The model under review builds one solid part; all positions refer to its coordinate system, in mm. A direction names the side the tool comes from. Round coordinates to 2 decimals unless told otherwise and drop trailing zeros. Order: outer loops, then holes, each group sorted by start corner. A loop starts at its lowest first (then second) coordinate and runs counter-clockwise, first axis right, second up.
Solid Edge part; units mm, degrees
sketch "Sketch1" plane through (0, 0, 0) normal (0, 0, 1) x (1, 0, 0)
  line L0 (-120, -60) -> (120, -60)
  line L1 (120, 120) -> (120, -60)
  line L2 (120, 120) -> (-120, 120)
  line L3 (-120, 120) -> (-120, -60)
extrude "Protrusion1" add sketch "Sketch1" along normal mid plane 50
fillet "Round_1" radius 30 4 edges at (-120, 120, 0) (-120, -60, 0) (120, -60, 0) (120, 120, 0)
hole "Hole_6" at (83, -30, -25) direction (0, 0, 1) diameter 4.917 depth 21
hole "Hole1" at (83, 30, -25) direction (0, 0, 1) diameter 4.917 depth 21
hole "Hole2" at (-83, 30, -25) direction (0, 0, 1) diameter 4.917 depth 21
hole "Hole3" at (-83, -30, -25) direction (0, 0, 1) diameter 4.917 depth 21
(1) Consider section B-B (x = 83). Write out the cut boundary in (y, z).
Data:
outline: (-60, -25) - (-32.46, -25) - (-32.46, -4) - (-27.54, -4) - (-27.54, -25) - (27.54, -25) - (27.54, -4) - (32.46, -4) - (32.46, -25) - (120, -25) - (120, 25) - (-60, 25) - close
(2) For faces 4 (the cylindrical face through (85.4, -30.53, -14.35)), 5 (the cylindrical face through (-111.445, 110.979, -0.35)), list the 3-axis set-ups (+Z, -Z, +X, -X, +Y, -Y) from which the entire face can be reached by the end or side of a thin tool; tool diameter is ignored.
Data:
face 4: -Z
face 5: +Z, -Z, -X, +Y
(3) Consider section D-D (y = -43). Write out the cut boundary in (x, z), and give its area (3 significant figures).
Data:
outline: (-117.04, -25) - (117.04, -25) - (117.04, 25) - (-117.04, 25) - close
area: 11,700 mm2
(4) Consider section C-C (z = -16). Write out the cut boundary in (x, y), and give its area (3 significant figures).
Data:
outline: (-120, -30) arc R30 ccw to (-90, -60) - (90, -60) arc R30 ccw to (120, -30) - (120, 90) arc R30 ccw to (90, 120) - (-90, 120) arc R30 ccw to (-120, 90) - close; hole circle Ø4.92 at (-83, -30); hole circle Ø4.92 at (-83, 30); hole circle Ø4.92 at (83, -30); hole circle Ø4.92 at (83, 30)
area: 42,400 mm2
(5) Consider section A-A (y = 30). Write out the cut boundary in (x, z), and give its area (3 significant figures).
Data:
outline: (-120, -25) - (-85.46, -25) - (-85.46, -4) - (-80.54, -4) - (-80.54, -25) - (80.54, -25) - (80.54, -4) - (85.46, -4) - (85.46, -25) - (120, -25) - (120, 25) - (-120, 25) - close
area: 11,800 mm2
(6) Draft analysis for pull direction Y (two halves, no side actions). For faces 1 (the flat face through (-83, 30, -4)), 2 (the flat face through (-2, 31, 25)), 3 (the cylindrical face through (-110.979, -51.445, -0.35)), state which applies: pulls with the +Y half, pulls with the -Y half, needs draft (parallel to the pull), parting line crosses it, or undercut.
Data:
face 1: undercut
face 2: needs draft
face 3: pulls with the -Y half
(7) Insertion check: pin 1 (8 mm diameter, centred on y = -41.5, z = -16, fed in from -X); pin 2 (1.5 mm diameter, centred on x = -82, y = -29, fed in from -Z). Each pin has a flat end and moves straight along its axis. Give the tip position at first contact, or say it passes through.
Data:
pin 1: stops at x = -119.05
pin 2: stops at z = -4
(8) To check wall thickness, follow probe 1 along Y at (x, z) = (-83, -11); probe 2 along X at (y, z) = (30, -13.75); probe 3 along X at (y, z) = (-43, -1.5). State the ranges of each line that lie inside material, in increasing order.
Data:
probe 1: y = -60 to -32.46, -27.54 to 27.54, 32.46 to 120
probe 2: x = -120 to -85.46, -80.54 to 80.54, 85.46 to 120
probe 3: x = -117.04 to 117.04
